Source: CAD feature listing. Evaluate the final solid. Frame: model axes, mm. A direction names the side the tool comes from. Give positions to 0.01 mm unless a question says otherwise; leave off trailing zeros. Write each loop counter-clockwise with the first axis right and the second up, starting at its lowest first coordinate (ties: lowest second). Pieces come first, ordered by that corner, then holes.
```python
from build123d import *

# Parameters (mm, degrees)
SKETCH1_W           = 120
SKETCH1_H           = 120
BOSS_EXTRUDE1_DEPTH = 3
SKETCH1_3_W         = 120
SKETCH1_3_H         = 120
SKETCH1_3_R         = 1.45
SKETCH1_3_W_2       = 100
SKETCH1_3_H_2       = 100
BOSS_EXTRUDE2_DEPTH = 10
BOSS_EXTRUDE3_START = 10
SKETCH5_W           = 120
SKETCH5_H           = 120
SKETCH5_R           = 1.45
SKETCH5_W_2         = 70.699570221
SKETCH5_H_2         = 15
SKETCH5_W_3         = 35
SKETCH5_H_3         = 50
SKETCH5_W_4         = 8.3907815
SKETCH5_H_4         = 37.710608616
BOSS_EXTRUDE3_DEPTH = 10


with BuildPart() as part:
    # Sketch1 → Boss-Extrude1 (new body)
    with BuildSketch(Plane(origin=(0, 0, 0), x_dir=(0, 1, 0), z_dir=(0, 0, 1))):
        Rectangle(SKETCH1_W, SKETCH1_H)
    extrude(amount=BOSS_EXTRUDE1_DEPTH)

    # Sketch1<3> → Boss-Extrude2 (add)
    # profile 1 of 3: a face of its own
    with BuildSketch(Plane(origin=(0, 0, 0), x_dir=(0, 1, 0), z_dir=(0, 0, 1))):
        Rectangle(SKETCH1_3_W, SKETCH1_3_H)
        with Locations(Location((-55, -55, 0), (0, 0, 270))):
            Circle(SKETCH1_3_R, mode=Mode.SUBTRACT)
        with Locations(Location((-55, 55, 0), (0, 0, 90))):
            Circle(SKETCH1_3_R, mode=Mode.SUBTRACT)
        with Locations(Location((55, -55, 0), (0, 0, 90))):
            Circle(SKETCH1_3_R, mode=Mode.SUBTRACT)
        with Locations(Location((55, 55, 0), (0, 0, 270))):
            Circle(SKETCH1_3_R, mode=Mode.SUBTRACT)
        Rectangle(SKETCH1_3_W_2, SKETCH1_3_H_2, mode=Mode.SUBTRACT)
    # profile 2 of 3: a face of its own
    with BuildSketch(Plane(origin=(0, 0, 0), x_dir=(0, 1, 0), z_dir=(0, 0, 1))):
        with Locations(Location((42.5, 1.5, 0), (0, 0, 270))):
            Circle(SKETCH1_3_R)
    # profile 3 of 3: a face of its own
    with BuildSketch(Plane(origin=(0, 0, 0), x_dir=(0, 1, 0), z_dir=(0, 0, 1))):
        with Locations(Location((-46, -46, 0), (0, 0, 270))):
            Circle(SKETCH1_3_R)
    extrude(amount=BOSS_EXTRUDE2_DEPTH)

    # Sketch5 → Boss-Extrude3 (add)
    with BuildSketch(Plane(origin=(0, 0, 0), x_dir=(0, 1, 0), z_dir=(0, 0, 1)).offset(BOSS_EXTRUDE3_START)):
        Rectangle(SKETCH5_W, SKETCH5_H)
        with Locations(Location((-55, -55, 0), (0, 0, 270))):
            Circle(SKETCH5_R, mode=Mode.SUBTRACT)
        with Locations(Location((-55, 55, 0), (0, 0, 270))):
            Circle(SKETCH5_R, mode=Mode.SUBTRACT)
        with Locations(Location((55, -55, 0), (0, 0, 270))):
            Circle(SKETCH5_R, mode=Mode.SUBTRACT)
        with Locations(Location((55, 55, 0), (0, 0, 270))):
            Circle(SKETCH5_R, mode=Mode.SUBTRACT)
        with Locations((6.34978511, 18.25)):
            Rectangle(SKETCH5_W_2, SKETCH5_H_2, mode=Mode.SUBTRACT)
        with Locations((-22.982605132, -22.59)):
            Rectangle(SKETCH5_W_3, SKETCH5_H_3, mode=Mode.SUBTRACT)
        with Locations((-1.13563625, -23.044910308)):
            Rectangle(SKETCH5_W_4, SKETCH5_H_4, mode=Mode.SUBTRACT)
        Polygon((27.574081379, -4.481691375), (28.750030367, -6.241709633), (28.748424488, -46.344003965), (26.988191952, -47.520096123), (12.885918621, -47.518308625), (11.709969633, -45.758290367), (11.711575511, -5.655996035), (13.471808048, -4.479903877), align=None, mode=Mode.SUBTRACT)
    extrude(amount=BOSS_EXTRUDE3_DEPTH)


solid = part.part
```
1. Cut plane C-C, the plane y = -10. Return the cut outline in (x, z).
2. Contact query for flat-ended pins moving along their axis: P1, Ø2.5, axis at x = 54.5, y = 54.5, coming from the +Z side; P2, Ø2.5, axis at x = 55, y = 55, coming from the +Z side. Output: stop coordinate, or through.
3. Cut plane B-B, the plane x = -43. Return the cut outline in (y, z), then the cut area to 3 significant figures.
4. Cut plane D-D, the plane x = 9. Return the cut outline in (y, z), then the cut area to 3 significant figures.
5. Line query: L1, parallel to X at y = 55, z = 13; L2, parallel to Z at x = -41, y = 34. Output: solid intervals per line, ascending.
6. Access query for faces 1 (the flat face through (1, 60, 10)), 2 (the flat face through (1, 50, 6)), 3 (the flat face through (-55, -55, 3)). Directions: +Z, -Z, +X, -X, +Y, -Y. A direction counts if a zero-diameter tool reaches every point of the face in a straight line with its end or side. Return the directions, or none.
7. Mould query, pull axis X, two halves, no side actions, for faces 4 (the cylindrical face through (-56.15, 54.12, 11.38)), 5 (the flat face through (-1, -1, 0)), 6 (the flat face through (-60, -1, 10)). Classes: +X half, -X half, draft (parallel to the pull), parting line (faces both ways), or undercut.
8. Cut plane A-A, the plane z = 8. Return the cut outline in (x, y).
Response values:
1. outline: (-60, 0) - (60, 0) - (60, 20) - (47.59, 20) - (47.59, 10) - (50, 10) - (50, 3) - (-50, 3) - (-50, 10) - (-25.75, 10) - (-25.75, 20) - (-60, 20) - close; (-10.75, 10) - (-2.41, 10) - (-2.41, 20) - (-10.75, 20) - close
2. P1: stops at z = 20
2. P2: stops at z = 3
3. outline: (-60, 0) - (60, 0) - (60, 20) - (-60, 20) - close; hole (-50, 3) - (50, 3) - (50, 10) - (-50, 10) - close
3. area: 1,700 mm2
4. outline: (-60, 0) - (60, 0) - (60, 20) - (28.75, 20) - (28.75, 10) - (50, 10) - (50, 3) - (-50, 3) - (-50, 10) - (-40.48, 10) - (-40.48, 20) - (-60, 20) - close; (-5.48, 10) - (-5.33, 10) - (-5.33, 20) - (-5.48, 20) - close; (3.06, 10) - (11.71, 10) - (11.71, 20) - (3.06, 20) - close
4. area: 1,100 mm2
5. L1: x = -60 to -56.45, -53.55 to 53.55, 56.45 to 60
5. L2: z = 0 to 3, 10 to 20
6. face 1: +Z, -Z, +X, -X, +Y
6. face 2: none
6. face 3: +Z
7. face 4: undercut
7. face 5: draft
7. face 6: -X half
8. outline: (-60, -60) - (60, -60) - (60, 60) - (-60, 60) - close; circle Ø2.9 at (-1.5, 42.5); circle Ø2.9 at (46, -46); hole circle Ø2.9 at (-55, -55); hole circle Ø2.9 at (-55, 55); hole (-50, -50) - (50, -50) - (50, 50) - (-50, 50) - close; hole circle Ø2.9 at (55, -55); hole circle Ø2.9 at (55, 55)
